```python
from build123d import *

# Parameters (mm, degrees)
F0_R     = 31.565
F1_DEPTH = 27.6
F2_R     = 2.5
F3_DEPTH = 9
F4_R     = 1.75
F5_DEPTH = 3
F6_R     = 1.5
F7_DEPTH = 5


with BuildPart() as f1:
    # F0 (on Top) → F1 (new body)
    with BuildSketch(Plane.XY):
        Circle(F0_R)
    extrude(amount=F1_DEPTH)

    # F2 (on face) → F3 (join)
    with BuildSketch(Plane(origin=(0, 0, 0), x_dir=(1, 0, 0), z_dir=(0, 0, -1))):
        Circle(F2_R)
    extrude(amount=F3_DEPTH)

    # F4 (on face) → F5 (join)
    with BuildSketch(Plane(origin=(0, 0, -9), x_dir=(1, 0, 0), z_dir=(0, 0, -1))):
        Circle(F4_R)
    extrude(amount=F5_DEPTH)

    # F6 (on face) → F7 (cut)
    with BuildSketch(Plane(origin=(0, 0, 0), x_dir=(1, 0, 0), z_dir=(0, 0, -1))):
        with Locations((0, 22)):
            Circle(F6_R)
        with Locations((0, -22)):
            Circle(F6_R)
        with Locations((-22, 0)):
            Circle(F6_R)
        with Locations((22, 0)):
            Circle(F6_R)
    extrude(amount=-F7_DEPTH, mode=Mode.SUBTRACT)


solid = f1.part
```
Geometry check sheet. Reference: the model listing, model coordinates, mm. A direction names the side the tool comes from. Coordinates: 2 decimals unless noted, no trailing zeros. Loops run counter-clockwise (first coordinate to the right, second up) from the corner with the lowest first, then second, coordinate; pieces in that order, holes last.
Item 1: Sectioned sample at C-C, the plane z = 11. Record the boundary of the cut face in (x, y) (3 decimals).
Item 2: Sectioned sample at A-A, the plane y = 0. Record the boundary of the cut face in (x, z) (3 decimals).
Item 3: Go/stop test with flat-tipped pins: pin 1 Ø3.5 at (x, y) = (0, -22) entering from -Z; pin 2 Ø8 at (x, z) = (-10.5, 5.5) entering from +Y; pin 3 Ø0.9 at (x, y) = (0.5, -22) entering from -Z. Record where each tip stops, or that it passes through.
Item 4: Thickness scan on line 1 (Y direction, x = 0, z = 1.25) (3 decimals); line 2 (Z direction, x = -4, y = 22.5); line 3 (X direction, y = 22, z = 1). Record the ranges inside material, lowest first.
Item 5: Access from +Z, -Z, +X, -X, +Y, -Y to the whole of each face (thin tool, end or side, straight path). Record for faces 1 (the face through (-25.049, -19.207, 13.607)), 2 (the face through (-0.195, -23.487, 2.465)).
Item 6: Release check for a two-part mould opening along Y. For faces 3 (the face through (1.617, 0.67, -10.479)), 4 (the face through (20.5, -0.07, 2.46)), 5 (the face through (-2, 1, -9)), 6 (the face through (-0.195, 20.513, 2.465)) record: released by +Y, released by -Y, zero draft, split by the parting line, or undercut.
Item 7: Sectioned sample at B-B, the plane x = -22. Record the boundary of the cut face in (y, z), then the cut area to 3 significant figures.
Check result:
1. outline: circle Ø63.13 at (0, 0)
2. outline: (-31.565, 0) - (-23.5, 0) - (-23.5, 5) - (-20.5, 5) - (-20.5, 0) - (-2.5, 0) - (-2.5, -9) - (-1.75, -9) - (-1.75, -12) - (1.75, -12) - (1.75, -9) - (2.5, -9) - (2.5, 0) - (20.5, 0) - (20.5, 5) - (23.5, 5) - (23.5, 0) - (31.565, 0) - (31.565, 27.6) - (-31.565, 27.6) - close
3. pin 1: stops at z = 0
3. pin 2: stops at y = 30.89
3. pin 3: stops at z = 5
4. line 1: y = -31.565 to -23.5, -20.5 to 20.5, 23.5 to 31.565
4. line 2: z = 0 to 27.6
4. line 3: x = -22.64 to -1.5, 1.5 to 22.64
5. face 1: +Z, -Z
5. face 2: -Z
6. face 3: split by the parting line
6. face 4: undercut
6. face 5: zero draft
6. face 6: undercut
7. outline: (-22.64, 0) - (-1.5, 0) - (-1.5, 5) - (1.5, 5) - (1.5, 0) - (22.64, 0) - (22.64, 27.6) - (-22.64, 27.6) - close
7. area: 1,230 mm2
